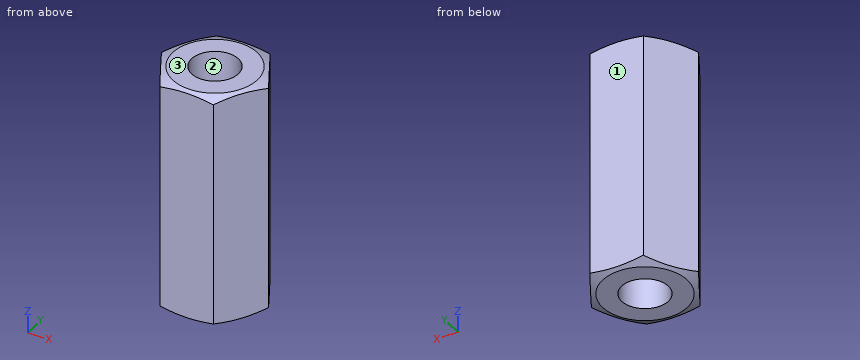
Autodesk Inventor part; units mm, degrees
ref_plane "YZ Plane" through (0, 0, 0) normal (1, 0, 0) x (0, 1, 0)
ref_plane "XZ Plane" through (0, 0, 0) normal (0, 1, 0) x (-1, 0, 0)
ref_plane "XY Plane" through (0, 0, 0) normal (0, 0, 1) x (1, 0, 0)
sketch "Skizze1" plane through (0, 0, 0) normal (0, 0, 1) x (1, 0, 0)
  line L0 (-3.2332, 0) -> (3.2332, 0) construction
  line L1 (0, -2.8) -> (0, 2.8) construction
  circle A0 centre (0, 0) radius 2 construction
  line L2 (1.1547, 2) -> (2.3094, 0)
  line L3 (2.3094, 0) -> (1.1547, -2)
  line L4 (1.1547, -2) -> (-1.1547, -2)
  line L5 (-1.1547, -2) -> (-2.3094, 0)
  line L6 (-2.3094, 0) -> (-1.1547, 2)
  line L7 (-1.1547, 2) -> (1.1547, 2)
  circle A1 centre (0, 0) radius 1
  point P0 (0, 2)
  dimension "d0" = 4
  dimension "d1" = 2
extrude "Extrusion1" add sketch "Skizze1" along normal blind 10
sketch "Skizze2" plane through (0, 0, 0) normal (0, 1, 0) x (-1, 0, 0)
  line L0 (1.1547, 10) -> (-1.1547, 10)
  line L1 (-1.1547, 10) -> (-2.3094, 10)
  line L2 (2.3094, 10) -> (1.1547, 10)
  line L3 (2.3094, 0) -> (1.1547, 0)
  line L4 (1.1547, 0) -> (-1.1547, 0)
  line L5 (-1.1547, 0) -> (-2.3094, 0)
  line L6 (-1.8094, 10) -> (-3.6188, 10)
  line L7 (-3.6188, 10) -> (-3.6188, 9.3414)
  line L8 (-3.6188, 9.3414) -> (-1.8094, 10)
  line L9 (-1.8094, 0) -> (-3.6188, 0.6586)
  line L10 (-3.6188, 0.6586) -> (-3.6188, 0)
  line L11 (-3.6188, 0) -> (-1.8094, 0)
  line L12 (0, -2) -> (0, 12)
  point P0 (0, 0)
  dimension "d4" = 20
  dimension "d5" = 0.5
revolve "Umdrehung1" cut sketch "Skizze2" angle 360 about axis through (0, 0, -10) along (0, 0, 1)
properties part number "Hex Spacer 10mm"
For this review, take the finished solid that the model builds, in its own axes (mm). Face numbers are marked on the shaded views. Give positions to 0.01 mm unless a question says otherwise; leave off trailing zeros. Loops run counter-clockwise (first coordinate to the right, second up) from the corner with the lowest first, then second, coordinate; pieces in that order, holes last. Notation, with made-up numbers: M 21,45.5 L 78,45.5 A6 cw 78,50.5 Z; hole C 49.25,64 d9. An arc over 180 degrees is marked long. One line per item, written item: value. Start each with the question number.
Q1. Add section A-A (x = 0). Give the boundary of the cut face in (y, z), and give its area (3 significant figures).
Q2. Draft analysis for pull direction Y (two halves, no side actions). For the marked faces 1, 2 and 3, state which applies: released by +Y, released by -Y, zero draft, split by the parting line, or undercut.
Q3. For L1, parallel to Y at x = 0, z = 2.75; L2, parallel to X at y = -0.15, z = 7.25; L3, parallel to X at y = 0.5, z = 1, list the stretches that pass through material, from the lowest coordinate up.
Q4. Clearance check with a flat-ended pin moving along its axis: pin 1 Ø1.5 at (y, z) = (0.5, 7) entering from -X. State where the tip first meets the part, or that it passes through.
Q5. Add section B-B (z = 3). Give the boundary of the cut face in (x, y).
Reply:
1. outline: M -2,0.07 L -1.81,0 L -1,0 L -1,10 L -1.81,10 L -2,9.93 Z; M 1,0 L 1.81,0 L 2,0.07 L 2,9.93 L 1.81,10 L 1,10 Z
1. area: 20.0 mm²
2. face 1: released by +Y
2. face 2: undercut
2. face 3: zero draft
3. L1: -2 to -1, 1 to 2
3. L2: -2.22 to -0.99, 0.99 to 2.22
3. L3: -2.02 to -0.87, 0.87 to 2.02
4. pin 1: x = -2.31
5. outline: M -2.31,0 L -1.15,-2 L 1.15,-2 L 2.31,0 L 1.15,2 L -1.15,2 Z; hole C 0,0 d2
